Work out the finished part from the listing and answer in its coordinate system (mm). Face numbers are marked on the shaded views. A direction names the side the tool comes from. Round coordinates to 2 decimals unless told otherwise and drop trailing zeros. Order: outer loops, then holes, each group sorted by start corner. A loop starts at its lowest first (then second) coordinate and runs counter-clockwise, first axis right, second up. Notation, with made-up numbers: (21.5, 83.5) - (65.5, 83.5) arc R21 cw to (65.5, 111.5) - close; hole circle Ø11 at (56, 57). An arc over 180 degrees is marked (long way). Use CSV: the item, a comma, the result in double quotes.
from build123d import *

# Parameters (mm, degrees)
SKETCH1_R           = 3.87
BOSS_EXTRUDE1_DEPTH = 11.89
SKETCH4_R           = 2.69
BOSS_EXTRUDE2_DEPTH = 2.78


with BuildPart() as part:
    # Sketch1 → Boss-Extrude1 (new body)
    with BuildSketch(Plane(origin=(0, 0, 0), x_dir=(1, 0, 0), z_dir=(0, 1, 0))):
        Circle(SKETCH1_R)
    extrude(amount=-BOSS_EXTRUDE1_DEPTH)

    # Sketch3 → Revolve1 (revolve)
    with BuildSketch(Plane.XY):
        with BuildLine():
            Line((0, 0), (0, 3.16))
            Line((0, 3.16), (3, 3.16))
            add(Edge.make_bspline(
                [(3, 3.16), (4.283639475, 3.024024765), (4.900890598, 1.632016655), (4.9, 0.5)],
                knots=[0, 0, 0, 0, 1, 1, 1, 1], degree=3))
            Line((4.9, 0.5), (4.9, 0))
            Line((4.9, 0), (0, 0))
        make_face()
    revolve(axis=Axis((0, 0, 0), (0, 1, 0)))

    # Sketch4 → Boss-Extrude2 (add)
    with BuildSketch(Plane(origin=(0, 3.16, 0), x_dir=(1, 0, 0), z_dir=(0, 1, 0))):
        Circle(SKETCH4_R)
    extrude(amount=BOSS_EXTRUDE2_DEPTH)


solid = part.part
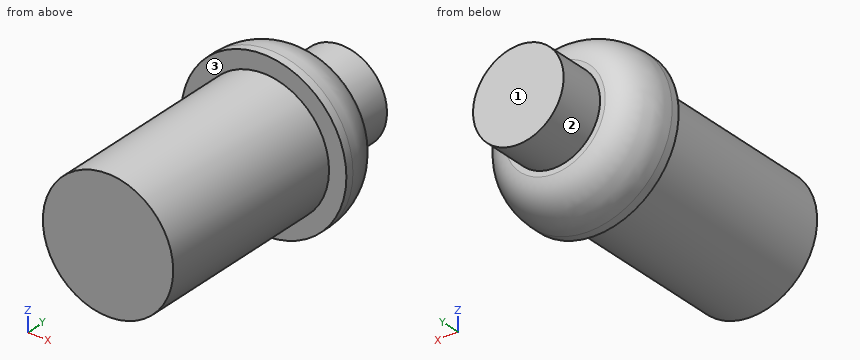
(1) For the marked faces 1, 2 and 3, determine the directions among +Z, -Z, +X, -X, +Y, -Y from which every point of the face is accessible in a straight line to the end or side of a thin tool.
Findings below:
face 1,"+Z, -Z, +X, -X, +Y"
face 2,"+Y"
face 3,"-Y"
(2) Each of these flat-tipped pins is pushed along its axis until it touches: pin 1 (4 mm diameter, centred on x = 2.5, y = -8, fed in from +Z); pin 2 (5 mm diameter, centred on x = 1, y = -3, fed in from -Z). Where does it stop, or does it pass through?
Findings below:
pin 1,"stops at z = 3.84"
pin 2,"stops at z = -3.87"
(3) Find the intervals of material crossed by L1, parallel to Y at x = -0.5, z = 4; L2, parallel to Y at x = -1.5, z = 3.25; L3, parallel to Z at x = 0, y = 5.25, in increasing order. Write a range as from..to.
Findings below:
L1,"y = 0..2.69"
L2,"y = -11.89..3"
L3,"z = -2.69..2.69"
(4) Find section A-A (y = -0.75). Determine the outline of the cut face in (x, z), and give its area (3 significant figures).
Findings below:
outline,"circle Ø7.74 at (0, 0)"
area,"47.1 mm²"
